```python
from build123d import *

# Parameters (mm, degrees)
F0_W     = 406.4
F0_H     = 228.6
F0_W_2   = 396.875
F0_H_2   = 219.075
F0_W_3   = 19.05
F0_R     = 4.7625
F0_W_4   = 12.7
F0_H_3   = 12.7
F0_R_2   = 2.5781
F1_DEPTH = 4.7752
F2_SIZE  = 3.81


with BuildPart() as f1:
    # F0 (on Top) → F1 (new body)
    with BuildSketch(Plane.XY):
        with Locations((-22.290767, 9.43711)):
            Rectangle(F0_W, F0_H)
        with Locations((-22.278067, 9.43711)):
            Rectangle(F0_W_2, F0_H_2, mode=Mode.SUBTRACT)
        with Locations((-235.015767, 9.43711)):
            Rectangle(F0_W_3, F0_H)
        with Locations((-235.015767, -85.81289)):
            Circle(F0_R, mode=Mode.SUBTRACT)
        with Locations((-235.015767, 104.68711)):
            Circle(F0_R, mode=Mode.SUBTRACT)
        with Locations((190.434233, 9.43711)):
            Rectangle(F0_W_3, F0_H)
        with Locations((190.434233, -85.81289)):
            Circle(F0_R, mode=Mode.SUBTRACT)
        with Locations((190.434233, 104.68711)):
            Circle(F0_R, mode=Mode.SUBTRACT)
        with Locations((-22.278067, 9.43711)):
            Rectangle(F0_W_2, F0_H_2)
        with Locations((-211.190567, -90.57539)):
            Rectangle(F0_W_4, F0_H_3, mode=Mode.SUBTRACT)
        with Locations((166.634433, -90.57539)):
            Rectangle(F0_W_4, F0_H_3, mode=Mode.SUBTRACT)
        with Locations((-211.190567, 109.44961)):
            Rectangle(F0_W_4, F0_H_3, mode=Mode.SUBTRACT)
        with Locations((166.634433, 109.44961)):
            Rectangle(F0_W_4, F0_H_3, mode=Mode.SUBTRACT)
        with Locations((-211.190567, 109.44961)):
            Rectangle(F0_W_4, F0_H_3)
        with Locations((-211.190567, 109.44961)):
            Circle(F0_R_2, mode=Mode.SUBTRACT)
        with Locations((-211.190567, -90.57539)):
            Rectangle(F0_W_4, F0_H_3)
        with Locations((-211.190567, -90.57539)):
            Circle(F0_R_2, mode=Mode.SUBTRACT)
        with Locations((166.634433, -90.57539)):
            Rectangle(F0_W_4, F0_H_3)
        with Locations((166.634433, -90.57539)):
            Circle(F0_R_2, mode=Mode.SUBTRACT)
        with Locations((166.634433, 109.44961)):
            Rectangle(F0_W_4, F0_H_3)
        with Locations((166.634433, 109.44961)):
            Circle(F0_R_2, mode=Mode.SUBTRACT)
    extrude(amount=F1_DEPTH)

    # F2
    f2_edges = [f1.edges().sort_by_distance(p)[0] for p in [
        (-213.768667, -90.57539, 0),
        (164.056333, -90.57539, 0),
        (164.056333, 109.44961, 0),
        (-213.768667, 109.44961, 0),
    ]]
    chamfer(f2_edges, length=F2_SIZE)


solid = f1.part
```
Source: CAD feature listing. Evaluate the final solid. Frame: model axes, mm. Round coordinates to 2 decimals unless told otherwise and drop trailing zeros. Put each result on its own line as item: value.
(1) Ray query, line 1 (X direction, y = -94, z = 0.45). Return the intervals inside material, ascending. Write a range as [from, to].
Solutions:
line 1: [-244.54, -216.04], [-206.34, 161.78], [171.49, 199.96]
(2) Pull-direction query (Y, two-part tool) for faces 1 (the face through (-25, 11, 4.775)), 2 (the face through (-208.59, 108.37, 3.57)); classes: released by +Y, released by -Y, zero draft, split by the parting line, or undercut.
Solutions:
face 1: zero draft
face 2: undercut
(3) First-contact query: pin 1 (8 mm diameter, centred on x = -211.19, y = -90.58, fed in from -Z); pin 2 (15 mm diameter, centred on x = -235.02, y = -85.81, fed in from +Z). Flat tips, straight axial feed; report the tip coordinate or a pass-through.
Solutions:
pin 1: z = 2.38
pin 2: z = 4.78
